Read the model definition and answer for the solid it produces. Units are mm, in the model's axes. Face numbers are marked on the shaded views. A direction names the side the tool comes from. Give positions to 0.01 mm unless a question says otherwise; leave off trailing zeros. Write each loop counter-clockwise with the first axis right and the second up, starting at its lowest first coordinate (ties: lowest second). Pieces come first, ordered by that corner, then holes. Notation, with made-up numbers: (-21.5, 32.25) -> (28.5, 32.25) arc R29 ccw to (28.5, 62.25) -> close; hole circle Ø10 at (16, 68). An arc over 180 degrees is marked (long way). Use a Markdown table: item, result.
from build123d import *

# Parameters (mm, degrees)
EXTRUDE_1_DEPTH     = 33.4
CUT_EXTRUDE_1_DEPTH = 1.2
CUT_EXTRUDE_2_DEPTH = 1.2
SKETCH_4_W          = 8.4
SKETCH_4_H          = 4.3
EXTRUDE_2_DEPTH     = 21.2
SKETCH_9_R          = 1.5
CUT_EXTRUDE_3_DEPTH = 3.1
SKETCH_10_R         = 5
CUT_EXTRUDE_4_DEPTH = 5.3
SKETCH_11_W         = 8.4
SKETCH_11_H         = 2
EXTRUDE_3_DEPTH     = 1


with BuildPart() as part:
    # 草图1 → 凸台-拉伸1 (new body)
    with BuildSketch(Plane.XY):
        Polygon((-16, 0), (-8, 0), (-7.7, 0.3), (7.7, 0.3), (8, 0), (16, 0), (16, 15.6), (7.6, 15.6), (7.6, 5.3), (-7.6, 5.3), (-7.6, 11.6), (-16, 11.6), align=None)
    extrude(amount=EXTRUDE_1_DEPTH)

    # 草图2 → 切除-拉伸1 (cut)
    with BuildSketch(Plane.XY):
        Polygon((-16, 0), (16, 0), (16, 15.6), (7.6, 15.6), (7.6, 11.6), (15.7, 11.6), (15.7, 0.3), (-15.7, 0.3), (-15.7, 11.1), (-7.6, 11.1), (-7.6, 11.6), (-16, 11.6), align=None)
    extrude(amount=CUT_EXTRUDE_1_DEPTH, mode=Mode.SUBTRACT)

    # 草图3 → 切除-拉伸2 (cut)
    with BuildSketch(Plane.XY.offset(33.4)):
        Polygon((-16, 0), (16, 0), (16, 15.6), (7.6, 15.6), (7.6, 11.1), (15.7, 11.1), (15.7, 0.3), (-15.7, 0.3), (-15.7, 11.1), (-7.6, 11.1), (-7.6, 11.6), (-16, 11.6), align=None)
    extrude(amount=-CUT_EXTRUDE_2_DEPTH, mode=Mode.SUBTRACT)

    # 草图4 → 凸台-拉伸2 (add)
    with BuildSketch(Plane.XY.offset(1.2)):
        with Locations((11.8, 13.45)):
            Rectangle(SKETCH_4_W, SKETCH_4_H)
    extrude(amount=-EXTRUDE_2_DEPTH)

    # 草图5 → 切除-旋转1 (revolve, cut)
    with BuildSketch(Plane.XY.offset(8.7)):
        Polygon((12, 4), (13.621, 4), (13.621, 0.379), (14, 0), (12, 0), align=None)
    revolve(axis=Axis((12, 0, 8.7), (0, 1, 0)), mode=Mode.SUBTRACT)

    # 草图6 → 切除-旋转2 (revolve, cut)
    with BuildSketch(Plane.XY.offset(8.7)):
        Polygon((-12, 4), (-10.379, 4), (-10.379, 0.379), (-10, 0), (-12, 0), align=None)
    revolve(axis=Axis((-12, 0, 8.7), (0, 1, 0)), mode=Mode.SUBTRACT)

    # 草图7 → 切除-旋转3 (revolve, cut)
    with BuildSketch(Plane.XY.offset(24.7)):
        Polygon((12, 4), (13.621, 4), (13.621, 0.379), (14, 0), (12, 0), align=None)
    revolve(axis=Axis((12, 0, 24.7), (0, 1, 0)), mode=Mode.SUBTRACT)

    # 草图8 → 切除-旋转4 (revolve, cut)
    with BuildSketch(Plane.XY.offset(24.7)):
        Polygon((-12, 4), (-10.379, 4), (-10.379, 0.379), (-10, 0), (-12, 0), align=None)
    revolve(axis=Axis((-12, 0, 24.7), (0, 1, 0)), mode=Mode.SUBTRACT)

    # 草图9 → 切除-拉伸3 (cut)
    with BuildSketch(Plane(origin=(0, 0.2, 0), x_dir=(1, 0, 0), z_dir=(0, 1, 0))):
        with Locations((0, -24.7)):
            Circle(SKETCH_9_R)
    extrude(amount=CUT_EXTRUDE_3_DEPTH, mode=Mode.SUBTRACT)

    # 草图10 → 切除-拉伸4 (cut)
    with BuildSketch(Plane(origin=(0, 0.2, 0), x_dir=(1, 0, 0), z_dir=(0, 1, 0))):
        with Locations((0, -9.2)):
            Circle(SKETCH_10_R)
    extrude(amount=CUT_EXTRUDE_4_DEPTH, mode=Mode.SUBTRACT)

    # 草图11 → 凸台-拉伸3 (add)
    with BuildSketch(Plane.XY.offset(-20)):
        with Locations((11.8, 16.6)):
            Rectangle(SKETCH_11_W, SKETCH_11_H)
    extrude(amount=EXTRUDE_3_DEPTH)


solid = part.part
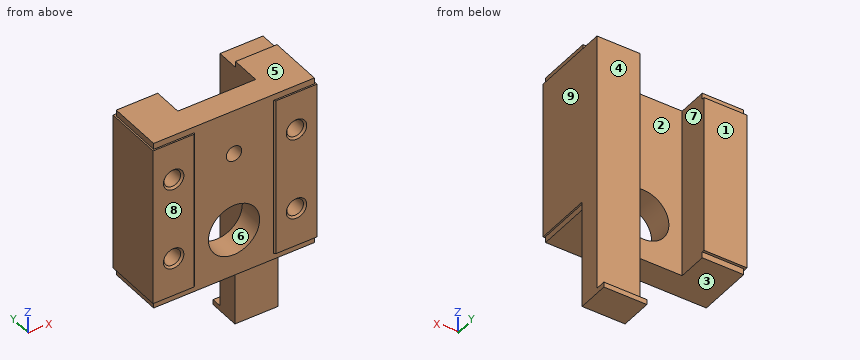
Item 1: A cutting plane is placed at C-C (x = 12). Give the vertices of the cut face in (y, z).
Return value:
| item | result |
|---|---|
| outline | (0, 1.2) -> (0.3, 1.2) -> (0.3, 0) -> (11.3, 0) -> (11.3, -20) -> (17.6, -20) -> (17.6, -19) -> (15.6, -19) -> (15.6, 32.2) -> (11.1, 32.2) -> (11.1, 33.4) -> (0.3, 33.4) -> (0.3, 32.2) -> (0, 32.2) -> (0, 26.7) -> (0.38, 26.32) -> (4, 26.32) -> (4, 23.08) -> (0.38, 23.08) -> (0, 22.7) -> (0, 10.7) -> (0.38, 10.32) -> (4, 10.32) -> (4, 7.08) -> (0.38, 7.08) -> (0, 6.7) -> close |
Item 2: A cutting plane is placed at B-B (z = 18). Give the vertices of the cut face in (x, y).
Return value:
| item | result |
|---|---|
| outline | (-16, 0) -> (-8, 0) -> (-7.7, 0.3) -> (7.7, 0.3) -> (8, 0) -> (16, 0) -> (16, 15.6) -> (7.6, 15.6) -> (7.6, 5.3) -> (-7.6, 5.3) -> (-7.6, 11.6) -> (-16, 11.6) -> close |
Item 3: A cutting plane is placed at A-A (x = 0). Give the vertices of the cut face in (y, z).
Return value:
| item | result |
|---|---|
| outline | (0.3, 0) -> (5.3, 0) -> (5.3, 4.2) -> (0.3, 4.2) -> close; (0.3, 14.2) -> (5.3, 14.2) -> (5.3, 33.4) -> (0.3, 33.4) -> (0.3, 26.2) -> (3.3, 26.2) -> (3.3, 23.2) -> (0.3, 23.2) -> close |
Item 4: Straight lines are drawn through the part: line 1 along Z through (x, y) = (12, 1.6); line 2 along Z through (x, y) = (0, 1); line 3 along X through (y, z) = (2.7, 24.7). For each, find the intervals that lie inside material, in ascending order. Write a range as [from, to].
Return value:
| item | result |
|---|---|
| line 1 | [0, 7.08], [10.32, 23.08], [26.32, 33.4] |
| line 2 | [0, 4.2], [14.2, 23.2], [26.2, 33.4] |
| line 3 | [-16, -13.62], [-10.38, -1.5], [1.5, 10.38], [13.62, 16] |
Item 5: A tool of negligible diameter and unlimited length cuts with its end or side. For the marked faces 1, 2, 3, 4 and 5, from which of +Z, -Z, +X, -X, +Y, -Y can it reach the whole face along a straight path? Write none if from no direction.
Return value:
| item | result |
|---|---|
| face 1 | +Z, -Z, -X, +Y |
| face 2 | +Z, -Z, +Y |
| face 3 | -Z, +X, -X, -Y |
| face 4 | +Z, +X, -X, +Y |
| face 5 | +Z, +X, -X, +Y, -Y |
Item 6: Each of these flat-tipped pins is pushed along its axis until it touches: P1, Ø6.5, axis at x = 10, z = -6, coming from the +Y side; P2, Ø3, axis at x = 12, z = 8.7, coming from the -Y side; P3, Ø1.3, axis at y = 7.5, z = 33, coming from the -X side. Where does it stop, or does it pass through?
Return value:
| item | result |
|---|---|
| P1 | y = 15.6 |
| P2 | y = 4 |
| P3 | x = -15.7 |
Item 7: For a pull along X with two mould halves and no side action, classify the marked faces 6, 7, 8 and 9 as +X half, -X half, draft (parallel to the pull), parting line (faces both ways), or undercut.
Return value:
| item | result |
|---|---|
| face 6 | undercut |
| face 7 | undercut |
| face 8 | draft |
| face 9 | +X half |
Item 8: A cutting plane is placed at D-D (y = 16.75). Give the vertices of the cut face in (x, z), then the cut area to 3 significant figures.
Return value:
| item | result |
|---|---|
| outline | (7.6, -20) -> (16, -20) -> (16, -19) -> (7.6, -19) -> close |
| area | 8.40 mm^2 |
